```python
from build123d import *

# Parameters (mm, degrees)
BOSS_EXTRUDE1_DEPTH = 25
SKETCH2_R           = 3
CUT_EXTRUDE1_DEPTH  = 25
SKETCH3_W           = 25
SKETCH3_H           = 25
BOSS_EXTRUDE2_DEPTH = 5
BOSS_EXTRUDE3_DEPTH = 192.5
BOSS_EXTRUDE4_START = 32.5
BOSS_EXTRUDE4_DEPTH = 32.5
LPATTERN4_COUNT     = 3
LPATTERN4_PITCH     = 80
CUT_EXTRUDE2_DEPTH  = 5


with BuildPart() as part:
    # Sketch1 → Boss-Extrude1 (new body)
    with BuildSketch(Plane(origin=(0, 0, 0), x_dir=(1, 0, 0), z_dir=(0, 1, 0))):
        with BuildLine():
            Line((-65.504745346, 11.478381524), (-65.504745346, -13.521618476))
            Line((-65.504745346, -13.521618476), (-75.504745346, -13.521618476))
            ThreePointArc((-75.504745346, -13.521618476), (-76.536999603, -1.021618476), (-75.504745346, 11.478381524))
            Line((-75.504745346, 11.478381524), (-65.504745346, 11.478381524))
        make_face()
    extrude(amount=BOSS_EXTRUDE1_DEPTH)

    # Sketch2 → Cut-Extrude1 (cut)
    with BuildSketch(Plane(origin=(-65.504745346, 0, 0), x_dir=(0, 0, -1), z_dir=(1, 0, 0))):
        with Locations((-1.021618476, 12.5)):
            Circle(SKETCH2_R)
    cut_extrude1 = extrude(amount=-CUT_EXTRUDE1_DEPTH, mode=Mode.SUBTRACT)

    # Sketch3 → Boss-Extrude2 (add)
    with BuildSketch(Plane(origin=(-65.504745346, 0, 0), x_dir=(0, 0, -1), z_dir=(1, 0, 0))):
        with Locations((-1.021618476, 12.5)):
            Rectangle(SKETCH3_W, SKETCH3_H)
        Polygon((5.906584755, 12.5), (2.442483139, 18.5), (-4.485720091, 18.5), (-7.949821706, 12.5), (-4.485720091, 6.5), (2.442483139, 6.5), align=None, mode=Mode.SUBTRACT)
    extrude(amount=BOSS_EXTRUDE2_DEPTH)

    # Sketch4 → Boss-Extrude3 (add)
    with BuildSketch(Plane(origin=(0, 25, 0), x_dir=(1, 0, 0), z_dir=(0, 1, 0))):
        with BuildLine():
            Line((-75.504745346, -13.521618476), (-60.504745346, -13.521618476))
            Line((-60.504745346, -13.521618476), (-60.504745346, 11.478381524))
            Line((-60.504745346, 11.478381524), (-75.504745346, 11.478381524))
            ThreePointArc((-75.504745346, 11.478381524), (-76.536999603, -1.021618476), (-75.504745346, -13.521618476))
        make_face()
    extrude(amount=BOSS_EXTRUDE3_DEPTH)

    # Sketch5 → Boss-Extrude4 (add)
    with BuildSketch(Plane.XZ.offset(BOSS_EXTRUDE4_START)):
        with BuildLine():
            Line((-75.504745346, 13.521618476), (-60.504745346, 13.521618476))
            Line((-60.504745346, 13.521618476), (-60.504745346, -11.478381524))
            Line((-60.504745346, -11.478381524), (-75.504745346, -11.478381524))
            ThreePointArc((-75.504745346, -11.478381524), (-76.536999603, 1.021618476), (-75.504745346, 13.521618476))
        make_face()
    extrude(amount=-BOSS_EXTRUDE4_DEPTH)

    # LPattern4: Cut-Extrude1 ×3
    with Locations(*[(0, i * LPATTERN4_PITCH, 0) for i in range(1, LPATTERN4_COUNT)]):
        add(cut_extrude1, mode=Mode.SUBTRACT)

    # Sketch6 → Cut-Extrude2 (cut)
    with BuildSketch(Plane(origin=(-60.504745346, 0, 0), x_dir=(0, 0, -1), z_dir=(1, 0, 0))):
        Polygon((5.906584755, 92.5), (2.442483139, 98.5), (-4.485720091, 98.5), (-7.949821706, 92.5), (-4.485720091, 86.5), (2.442483139, 86.5), align=None)
        Polygon((5.906584755, 172.5), (2.442483139, 178.5), (-4.485720091, 178.5), (-7.949821706, 172.5), (-4.485720091, 166.5), (2.442483139, 166.5), align=None)
    extrude(amount=-CUT_EXTRUDE2_DEPTH, mode=Mode.SUBTRACT)


solid = part.part
```
Input: part model. Units: mm. Frame: model coordinates. A direction names the side the tool comes from. Coordinates: 2 decimals unless noted, no trailing zeros. Write each loop counter-clockwise with the first axis right and the second up, starting at its lowest first coordinate (ties: lowest second). Pieces come first, ordered by that corner, then holes. Notation, with made-up numbers: (18.5, -18.5) -> (58.5, -18.5) arc R7 cw to (58.5, -8.5) -> close; hole circle Ø10 at (-13, -25). An arc over 180 degrees is marked (long way). Answer as a JSON object with one key per item and string values.
1. Section B-B on y = 142. Return the cut outline in (x, z).
Result set:
{"outline": "(-75.5, -11.48) -> (-60.5, -11.48) -> (-60.5, 13.52) -> (-75.5, 13.52) arc R76.2 ccw to start"}
2. Material intervals for line 1 (Y direction, x = -75, z = 2.5); line 2 (Z direction, x = -68, y = 172.5); line 3 (Y direction, x = -71.5, z = -0.25), sorted ascending. Write a range as from..to.
Result set:
{"line 1": "y = -32.5..9.89, 15.11..89.89, 95.11..169.89, 175.11..217.5", "line 2": "z = -11.48..-1.98, 4.02..13.52", "line 3": "y = -32.5..9.78, 15.22..89.78, 95.22..169.78, 175.22..217.5"}
3. Mould query, pull axis Y, two halves, no side actions, for faces 1 (the face through (-68, -32.5, 1)), 2 (the face through (-69, 217.5, 1)), 3 (the face through (-63, 166.5, 1)). Classes: released by +Y, released by -Y, zero draft, split by the parting line, or undercut.
Result set:
{"face 1": "released by -Y", "face 2": "released by +Y", "face 3": "undercut"}
4. Access query for faces 4 (the face through (-70.945, 175.474, 1.412)), 5 (the face through (-62.97, 175.542, 6.194)). Directions: +Z, -Z, +X, -X, +Y, -Y. A direction counts if a zero-diameter tool reaches every point of the face in a straight line with its end or side. Return the directions, or none.
Result set:
{"face 4": "+X, -X", "face 5": "+X"}
5. Section A-A on z = 2. Return the cut outline in (x, y), then the cut area to 3 significant figures.
Result set:
{"outline": "(-76.53, -32.5) -> (-60.5, -32.5) -> (-60.5, 6.5) -> (-65.5, 6.5) -> (-65.5, 9.66) -> (-76.53, 9.66) -> close; (-76.53, 15.34) -> (-65.5, 15.34) -> (-65.5, 18.5) -> (-60.5, 18.5) -> (-60.5, 86.5) -> (-65.5, 86.5) -> (-65.5, 89.66) -> (-76.53, 89.66) -> close; (-76.53, 95.34) -> (-65.5, 95.34) -> (-65.5, 98.5) -> (-60.5, 98.5) -> (-60.5, 166.5) -> (-65.5, 166.5) -> (-65.5, 169.66) -> (-76.53, 169.66) -> close; (-76.53, 175.34) -> (-65.5, 175.34) -> (-65.5, 178.5) -> (-60.5, 178.5) -> (-60.5, 217.5) -> (-76.53, 217.5) -> close", "area": "3,640 mm2"}
6. First-contact query: P1, Ø7, axis at y = 92.5, z = 1.02, coming from the +X side. Flat tip, straight axial feed; report the tip coordinate or a pass-through.
Result set:
{"P1": "stops at x = -65.5"}
